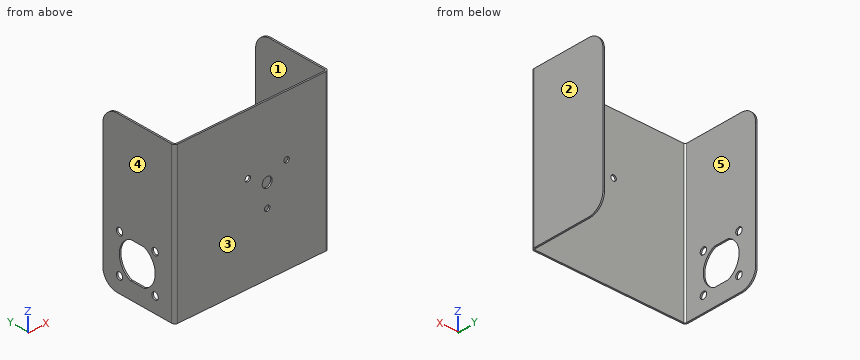
from build123d import *

# Parameters (mm, degrees)
SKETCH1_W                    = 100
SKETCH1_H                    = 100
BASE_FLANGE1_DEPTH           = 1
EDGE_FLANGE1_STRIP_W         = 6
EDGE_FLANGE1_STRIP_H         = 1
EDGE_FLANGE1_STRIP_CUT_DEPTH = 100
EDGE_FLANGE1_DEPTH           = 100
EDGE_FLANGE2_STRIP_W         = 6
EDGE_FLANGE2_STRIP_H         = 1
EDGE_FLANGE2_STRIP_CUT_DEPTH = 100
EDGE_FLANGE2_DEPTH           = 100
FILLET1_R                    = 10
SKETCH12_R                   = 2.25
CUT_EXTRUDE1_DEPTH           = 10
SKETCH13_R                   = 3.25
SKETCH13_R_2                 = 1.75
CUT_EXTRUDE2_DEPTH           = 8


# Sheet-metal steps are written as plain solids
with BuildPart() as part:
    # Sketch1 → Base-Flange1 (new body)
    with BuildSketch(Plane(origin=(0, 0, 0), x_dir=(1, 0, 0), z_dir=(0, 1, 0))):
        with Locations((50, 50)):
            Rectangle(SKETCH1_W, SKETCH1_H)
    extrude(amount=-BASE_FLANGE1_DEPTH)

    # Edge-Flange1 strip (across the edge) → Edge-Flange1 strip cut (cut)
    with BuildSketch(Plane(origin=(100, 0, 0), x_dir=(-1, 0, 0), z_dir=(0, 0, -1))):
        with Locations((-1, -0.5)):
            Rectangle(EDGE_FLANGE1_STRIP_W, EDGE_FLANGE1_STRIP_H)
    extrude(amount=EDGE_FLANGE1_STRIP_CUT_DEPTH, mode=Mode.SUBTRACT)

    # Edge-Flange1 section (across the edge) → Edge-Flange1 (add)
    with BuildSketch(Plane(origin=(100, 0, 0), x_dir=(-1, 0, 0), z_dir=(0, 0, -1))):
        with BuildLine():
            Line((0, 1), (0, 49))
            Line((0, 49), (1, 49))
            Line((1, 49), (1, 1))
            ThreePointArc((1, 1), (1.292893219, 0.292893219), (2, 0))
            Line((2, 0), (2, -1))
            ThreePointArc((2, -1), (0.585786438, -0.414213562), (0, 1))
        make_face()
    extrude(amount=EDGE_FLANGE1_DEPTH)

    # Edge-Flange2 strip (across the edge) → Edge-Flange2 strip cut (cut)
    with BuildSketch(Plane.XY.offset(-100)):
        with Locations((-1, -0.5)):
            Rectangle(EDGE_FLANGE2_STRIP_W, EDGE_FLANGE2_STRIP_H)
    extrude(amount=EDGE_FLANGE2_STRIP_CUT_DEPTH, mode=Mode.SUBTRACT)

    # Edge-Flange2 section (across the edge) → Edge-Flange2 (add)
    with BuildSketch(Plane.XY.offset(-100)):
        with BuildLine():
            Line((0, 1), (0, 49))
            Line((0, 49), (1, 49))
            Line((1, 49), (1, 1))
            ThreePointArc((1, 1), (1.292893219, 0.292893219), (2, 0))
            Line((2, 0), (2, -1))
            ThreePointArc((2, -1), (0.585786438, -0.414213562), (0, 1))
        make_face()
    extrude(amount=EDGE_FLANGE2_DEPTH)

    # Fillet1
    fillet1_edges = [part.edges().sort_by_distance(p)[0] for p in [
        (99.5, 49, 0),
        (99.5, 49, -100),
        (0.5, 49, -100),
        (0.5, 49, 0),
    ]]
    fillet(fillet1_edges, radius=FILLET1_R)

    # Sketch12 → Cut-Extrude1 (cut)
    with BuildSketch(Plane(origin=(-1, -31.373526732, -102.532454166), x_dir=(0, 0, 1), z_dir=(-1, 0, 0))):
        with BuildLine():
            ThreePointArc((36.332454166, 61.272506218), (24.832454166, 68.873526732), (13.332454166, 61.272506218))
            Line((13.332454166, 61.272506218), (13.332454166, 51.474547246))
            ThreePointArc((13.332454166, 51.474547246), (24.832454166, 43.873526732), (36.332454166, 51.474547246))
            Line((36.332454166, 51.474547246), (36.332454166, 61.272506218))
        make_face()
        with Locations(Location((12.458085495, 68.747895403, 0), (0, 0, 90))):
            Circle(SKETCH12_R)
        with Locations(Location((37.206822836, 68.747895403, 0), (0, 0, 90))):
            Circle(SKETCH12_R)
        with Locations(Location((37.206822836, 43.999158061, 0), (0, 0, 90))):
            Circle(SKETCH12_R)
        with Locations(Location((12.458085495, 43.999158061, 0), (0, 0, 90))):
            Circle(SKETCH12_R)
    extrude(amount=-CUT_EXTRUDE1_DEPTH, mode=Mode.SUBTRACT)

    # Sketch13 → Cut-Extrude2 (cut)
    with BuildSketch(Plane(origin=(17.313345769, -1, -102.532454166), x_dir=(1, 0, 0), z_dir=(0, -1, 0))):
        with Locations(Location((42.686654231, 56.832454166, 0), (0, 0, 270))):
            Circle(SKETCH13_R)
        with Locations(Location((30.129285876, 64.082454166, 0), (0, 0, 270))):
            Circle(SKETCH13_R_2)
        with Locations(Location((55.244022586, 64.082454166, 0), (0, 0, 270))):
            Circle(SKETCH13_R_2)
        with Locations(Location((42.686654231, 42.332454166, 0), (0, 0, 270))):
            Circle(SKETCH13_R_2)
    extrude(amount=-CUT_EXTRUDE2_DEPTH, mode=Mode.SUBTRACT)


solid = part.part
Check sheet for the modelled part. Datum: model origin and axes. Units: mm. Face numbers are marked on the shaded views. A direction names the side the tool comes from. Give positions to 0.01 mm unless a question says otherwise; leave off trailing zeros. Loops run counter-clockwise (first coordinate to the right, second up) from the corner with the lowest first, then second, coordinate; pieces in that order, holes last. Notation, with made-up numbers: M -1.75,55.5 L 33.25,55.5 A16 ccw 33.25,83.5 Z; hole C 56.25,58 d11. An arc over 180 degrees is marked long. Answer as a JSON object with one key per item and string values. Group by question number.
Q1. Material ranges on line 1 along X through (y, z) = (42, -85.5); line 2 along Y through (x, z) = (89.5, -51.5); line 3 along X through (y, z) = (-0.45, -60.2), recorded low to high. Write a range as [from, to].
Q2. Cross-section at C-C on y = 24. Record the cut outline in (x, z), then the cut area to 3 significant figures.
Q3. Cross-section at B-B on y = 5.5. Record the cut outline in (x, z).
Q4. Go/stop test with flat-tipped pins: P1, Ø2.5, axis at y = 37.37, z = -65.33, coming from the -X side; P2, Ø8.5, axis at x = 60, z = -45.7, coming from the -Y side; P3, Ø1.5, axis at x = 18, z = -18, coming from the +Y side. Record where each tip stops, or that it passes through.
Q5. Cross-section at D-D on z = -60.2. Record the cut outline in (x, y), then the cut area to 3 significant figures.
Q6. Release check for a two-part mould opening along X. For the marked faces 1, 2 and 3 record: released by +X, released by -X, zero draft, split by the parting line, or undercut.
Q7. Access from +Z, -Z, +X, -X, +Y, -Y to the whole of each face (thin tool, end or side, straight path). Record for the marked faces 4 and 5.
Q8. Cross-section at A-A on z = -38.45. Record the cut outline in (x, y).
Evaluation:
{
 "1": {"line 1": "x = [0, 1], [99, 100]", "line 2": "y = [-1, 0]", "line 3": "x = [0.62, 58.25], [61.75, 99.38]"},
 "2": {"outline": "M 0,-100 L 1,-100 L 1,-89.2 L 0,-89.2 Z; M 0,-66.2 L 1,-66.2 L 1,0 L 0,0 Z; M 99,-100 L 100,-100 L 100,0 L 99,0 Z", "area": "177 mm2"},
 "3": {"outline": "M 0,-100 L 1,-100 L 1,0 L 0,0 Z; M 99,-100 L 100,-100 L 100,0 L 99,0 Z"},
 "4": {"P1": "stops at x = 99", "P2": "stops at y = -1", "P3": "stops at y = 0"},
 "5": {"outline": "M 0,1 A2 ccw 2,-1 L 58.25,-1 L 58.25,0 L 2,0 A1 cw 1,1 L 1,49 L 0,49 Z; M 61.75,-1 L 98,-1 A2 ccw 100,1 L 100,49 L 99,49 L 99,1 A1 cw 98,0 L 61.75,0 Z", "area": "193 mm2"},
 "6": {"face 1": "undercut", "face 2": "released by +X", "face 3": "zero draft"},
 "7": {"face 4": "+Z, -Z, -X, +Y, -Y", "face 5": "+Z, -Z, +Y"},
 "8": {"outline": "M 0,1 A2 ccw 2,-1 L 45.69,-1 L 45.69,0 L 2,0 A1 cw 1,1 L 1,49 L 0,49 Z; M 49.19,-1 L 70.81,-1 L 70.81,0 L 49.19,0 Z; M 74.31,-1 L 98,-1 A2 ccw 100,1 L 100,49 L 99,49 L 99,1 A1 cw 98,0 L 74.31,0 Z"}
}
